Geometry: final body of the model. Coordinates: model frame, mm. A direction names the side the tool comes from. Give positions to 0.01 mm unless a question says otherwise; leave off trailing zeros. Loops run counter-clockwise (first coordinate to the right, second up) from the corner with the lowest first, then second, coordinate; pieces in that order, holes last. Notation, with made-up numbers: (-32, 44) - (-8, 44) arc R19 ccw to (-8, 68) - close; hole circle Ø5 at (-29.5, 88). An arc over 180 degrees is marked (long way). Use one line per item in the form item = value.
```python
from build123d import *

# Parameters (mm, degrees)
SKETCH1_R           = 5.5
SKETCH1_R_2         = 1.4
BOSS_EXTRUDE1_DEPTH = 5
SKETCH2_R           = 2.65
CUT_EXTRUDE1_DEPTH  = 2.5
SKETCH3_R           = 4.4
CUT_EXTRUDE2_DEPTH  = 3


with BuildPart() as part:
    # Sketch1 → Boss-Extrude1 (new body)
    with BuildSketch(Plane.XY):
        with BuildLine():
            ThreePointArc((-3.788390561, 28.237877779), (0, 30.4), (3.788390561, 28.237877779))
            ThreePointArc((3.788390561, 28.237877779), (17.5, 13), (36.048454046, 4.273259191))
            ThreePointArc((36.048454046, 4.273259191), (39.4, 0), (36.048454046, -4.273259191))
            ThreePointArc((36.048454046, -4.273259191), (17.5, -13), (3.788390561, -28.237877779))
            ThreePointArc((3.788390561, -28.237877779), (0, -30.4), (-3.788390561, -28.237877779))
            ThreePointArc((-3.788390561, -28.237877779), (-17.5, -13), (-36.048454046, -4.273259191))
            ThreePointArc((-36.048454046, -4.273259191), (-39.4, 0), (-36.048454046, 4.273259191))
            ThreePointArc((-36.048454046, 4.273259191), (-17.5, 13), (-3.788390561, 28.237877779))
        make_face()
        Circle(SKETCH1_R, mode=Mode.SUBTRACT)
        with Locations((0, 10)):
            Circle(SKETCH1_R_2, mode=Mode.SUBTRACT)
        with Locations((10, 0)):
            Circle(SKETCH1_R_2, mode=Mode.SUBTRACT)
        with Locations((0, -10)):
            Circle(SKETCH1_R_2, mode=Mode.SUBTRACT)
        with Locations((-10, 0)):
            Circle(SKETCH1_R_2, mode=Mode.SUBTRACT)
        with Locations((35, 0)):
            Circle(SKETCH1_R_2, mode=Mode.SUBTRACT)
        with Locations((0, 26)):
            Circle(SKETCH1_R_2, mode=Mode.SUBTRACT)
        with Locations((0, -26)):
            Circle(SKETCH1_R_2, mode=Mode.SUBTRACT)
        with Locations((-35, 0)):
            Circle(SKETCH1_R_2, mode=Mode.SUBTRACT)
    extrude(amount=BOSS_EXTRUDE1_DEPTH)

    # Sketch2 → Cut-Extrude1 (cut)
    with BuildSketch(Plane.XY.offset(5)):
        with Locations((0, 10)):
            Circle(SKETCH2_R)
        with Locations((10, 0)):
            Circle(SKETCH2_R)
        with Locations((0, -10)):
            Circle(SKETCH2_R)
        with Locations((-10, 0)):
            Circle(SKETCH2_R)
    extrude(amount=-CUT_EXTRUDE1_DEPTH, mode=Mode.SUBTRACT)

    # Sketch3 → Cut-Extrude2 (cut)
    with BuildSketch(Plane(origin=(0, 0, 0), x_dir=(-1, 0, 0), z_dir=(0, 0, -1))):
        with Locations((0, 26)):
            Circle(SKETCH3_R)
        with Locations((35, 0)):
            Circle(SKETCH3_R)
        with Locations((0, -26)):
            Circle(SKETCH3_R)
        with Locations((-35, 0)):
            Circle(SKETCH3_R)
    extrude(amount=-CUT_EXTRUDE2_DEPTH, mode=Mode.SUBTRACT)


solid = part.part
```
(1) Access query for faces 5 (the face through (0.75, 11.18, 1.23)), 6 (the face through (-12.647, 0.117, 3.768)). Directions: +Z, -Z, +X, -X, +Y, -Y. A direction counts if a zero-diameter tool reaches every point of the face in a straight line with its end or side. Return the directions, or none.
Solution:
face_5 = +Z, -Z
face_6 = +Z
(2) Cut plane D-D (x = -15). Return the cut outline in (y, z), plus the area to 3 significant figures.
Solution:
outline = (-14.98, 0) - (14.98, 0) - (14.98, 5) - (-14.98, 5) - close
area = 150 mm2
(3) Cut plane C-C (y = 0). Give the number of separate pieces and of enclosed holes in the cut face, plus the area to 4 significant figures.
Solution:
separate_pieces = 6
enclosed_holes = 0
area = 234.5 mm2
(4) Material intervals for L1, parallel to Y at x = 0, z = 2.4; L2, parallel to Y at x = 0, z = 3.55; L3, parallel to Y at x = 1, z = 1.9, sorted ascending. Write a range as from..to.
Solution:
L1 = -21.6..-11.4, -8.6..-5.5, 5.5..8.6, 11.4..21.6
L2 = -30.4..-27.4, -24.6..-12.65, -7.35..-5.5, 5.5..7.35, 12.65..24.6, 27.4..30.4
L3 = -21.72..-10.98, -9.02..-5.41, 5.41..9.02, 10.98..21.72
(5) Cut plane B-B (x = 35). Return the cut outline in (y, z).
Solution:
outline = (-4.54, 0) - (-4.4, 0) - (-4.4, 3) - (-1.4, 3) - (-1.4, 5) - (-4.54, 5) - close; (1.4, 3) - (4.4, 3) - (4.4, 0) - (4.54, 0) - (4.54, 5) - (1.4, 5) - close
(6) Pull-direction query (X, two-part tool) for faces 1 (the face through (-39.4, -0.1, 4)), 2 (the face through (1.1, -11.1, 2.5)), 3 (the face through (-11.4, 0.06, 1.23)), 4 (the face through (1, -6, 5)); classes: released by +X, released by -X, zero draft, split by the parting line, or undercut.
Solution:
face_1 = released by -X
face_2 = undercut
face_3 = undercut
face_4 = zero draft
(7) Pin query (flat end, axial travel): P1, Ø3.5, axis at x = 0, y = -10, coming from the +Z side; P2, Ø3, axis at y = 17.5, z = 1.5, coming from the +X side; P3, Ø2, axis at x = -11, z = 3, coming from the -Y side. Return the tip coordinate at first contact, or that it passes through.
Solution:
P1 = 2.5
P2 = 13.83
P3 = -19.8
(8) Cut plane A-A (y = -10). Return the cut outline in (x, z), plus the area to 3 significant figures.
Solution:
outline = (-22.01, 0) - (-1.4, 0) - (-1.4, 2.5) - (-2.65, 2.5) - (-2.65, 5) - (-22.01, 5) - close; (1.4, 0) - (22.01, 0) - (22.01, 5) - (2.65, 5) - (2.65, 2.5) - (1.4, 2.5) - close
area = 200 mm2
